Geometry check sheet. Reference: the model listing, model coordinates, mm. Face numbers are marked on the shaded views. A direction names the side the tool comes from. Coordinates: 2 decimals unless noted, no trailing zeros. Loops run counter-clockwise (first coordinate to the right, second up) from the corner with the lowest first, then second, coordinate; pieces in that order, holes last.
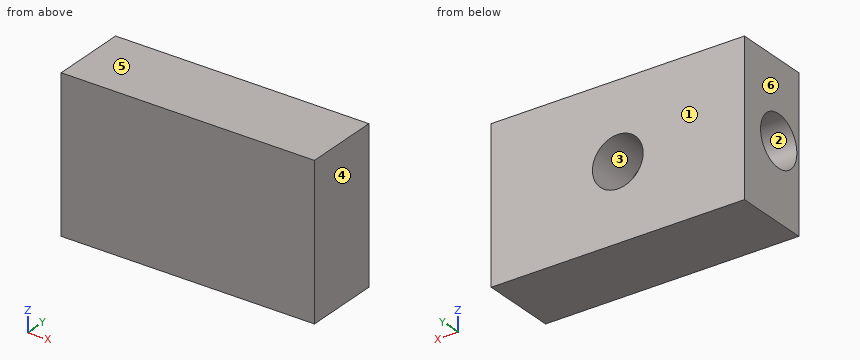
from build123d import *

# Parameters (mm, degrees)
F0_W     = 127
F0_H     = 76.2
F2_DEPTH = 38.1
F1_R     = 12.7
F3_DEPTH = 25.4
F4_R     = 12.7
F5_DEPTH = 76.2


with BuildPart() as f2:
    # F0 (on Front) → F2 (new body)
    with BuildSketch(Plane.XZ):
        with Locations((2e-06, 0.01443)):
            Rectangle(F0_W, F0_H)
    extrude(amount=F2_DEPTH)

    # F1 (on Front) → F3 (cut)
    with BuildSketch(Plane.XZ):
        Circle(F1_R)
    extrude(amount=F3_DEPTH, mode=Mode.SUBTRACT)

    # F4 (on Right) → F5 (cut)
    with BuildSketch(Plane.YZ):
        with Locations((-23.99939, 0)):
            Circle(F4_R)
    extrude(amount=-F5_DEPTH, mode=Mode.SUBTRACT)


solid = f2.part
1) Access from +Z, -Z, +X, -X, +Y, -Y to the whole of each face (thin tool, end or side, straight path). Record for the marked faces 1 and 2.
Data:
face 1: +Z, -Z, +X, -X, +Y
face 2: -X
2) Section check B-B on y = -7.5. Record the cut outline in (x, z), and give its area (3 significant figures).
Data:
outline: (-63.5, -38.09) - (63.5, -38.09) - (63.5, 38.11) - (-63.5, 38.11) - close; hole circle Ø25.4 at (0, 0)
area: 9,170 mm2
3) Section check A-A on z = 0. Record the cut outline in (x, y), and give its area (3 significant figures).
Data:
outline: (-63.5, -38.1) - (63.5, -38.1) - (63.5, 0) - (12.7, 0) - (12.7, -25.4) - (0, -25.4) - (0, -36.7) - (-63.5, -36.7) - close; (-63.5, -11.3) - (-12.7, -11.3) - (-12.7, 0) - (-63.5, 0) - close
area: 2,760 mm2
4) Material ranges on probe 1 along Z at (x, y) = (0, -8.5); probe 2 along Y at (x, z) = (-34, 0); probe 3 along Y at (x, z) = (1.5, -5), recorded low to high.
Data:
probe 1: z = -38.09 to -12.7, 12.7 to 38.11
probe 2: y = -38.1 to -36.7, -11.3 to 0
probe 3: y = -38.1 to -25.4
5) Section check D-D on y = -32. Record the cut outline in (x, z).
Data:
outline: (-63.5, -38.09) - (63.5, -38.09) - (63.5, 38.11) - (-63.5, 38.11) - (-63.5, 9.86) - (0, 9.86) - (0, -9.86) - (-63.5, -9.86) - close
6) Section check C-C on x = -37.5. Record the cut outline in (y, z).
Data:
outline: (-38.1, -38.09) - (0, -38.09) - (0, 38.11) - (-38.1, 38.11) - close; hole circle Ø25.4 at (-24, 0)
7) Depth check by flat-ended pin: pin 1 (3.5 mm diameter, centred on y = -32.5, z = 1.5, fed in from -X); pin 2 (4 mm diameter, centred on x = 7, z = 3, fed in from +Y). Enter the tip coordinate at first touch or a pass-through.
Data:
pin 1: stops at x = 0
pin 2: stops at y = -25.4
8) Mould release check, pull along X, two halves, no side actions. Record for the marked faces 3, 4, 5 and 6: +X half, -X half, draft (parallel to the pull), parting line (faces both ways), or undercut.
Data:
face 3: undercut
face 4: +X half
face 5: draft
face 6: -X half
